Can you work these out from the model? Positions are in its coordinate system, mm. A direction names the side the tool comes from. Give positions to 0.01 mm unless a question says otherwise; leave off trailing zeros. Loops run counter-clockwise (first coordinate to the right, second up) from the corner with the lowest first, then second, coordinate; pieces in that order, holes last. Notation, with made-up numbers: M -38,46 L -3,46 A9 cw -3,54 Z; hole C -1.75,63 d11. An arc over 180 degrees is marked long. One line per item, written item: value. Start each with the question number.
from build123d import *

# Parameters (mm, degrees)
PAD_DEPTH    = 0.8
PAD001_DEPTH = 10
SKETCH003_R  = 3
PAD002_DEPTH = 6
POCKET_DEPTH = 5


with BuildPart() as part:
    # Sketch → Pad (new body)
    with BuildSketch(Plane.XZ):
        with BuildLine():
            Line((-25.5, 14.5), (-25.5, 48))
            ThreePointArc((-21.5, 52), (-24.328427, 50.828427), (-25.5, 48))
            Line((-21.5, 52), (21.5, 52))
            ThreePointArc((25.5, 48), (24.328427, 50.828427), (21.5, 52))
            Line((25.5, 48), (25.5, 14.5))
            Line((25.5, 14.5), (15.5, 14.5))
            Line((15.5, 14.5), (15.5, 24))
            Line((15.5, 24), (-15.5, 24))
            Line((-15.5, 24), (-15.5, 14.5))
            Line((-15.5, 14.5), (-25.5, 14.5))
        make_face()
    extrude(amount=PAD_DEPTH)

    # Sketch001 → Pad001 (join, symmetric)
    with BuildSketch(Plane.YZ):
        Polygon((-2, 24), (-9.7, 31.7), (-9.7, 32.5), (0, 32.5), (0, 24), align=None)
    extrude(amount=PAD001_DEPTH, both=True)

    # Sketch003 (on Face12 of Pad001) → Pad002 (join)
    with BuildSketch(Plane(origin=(0, 0, 32.5), x_dir=(-1, 0, 0), z_dir=(0, 0, 1))):
        with Locations((0, 5.5)):
            Circle(SKETCH003_R)
    extrude(amount=-PAD002_DEPTH)

    # Sketch004 (on Face5 of Pad002) → Pocket (cut)
    with BuildSketch(Plane.XZ.offset(0.8)):
        with BuildLine():
            Line((-12, 38.8), (-12, 46.8))
            Line((-12, 46.8), (-8, 46.8))
            Line((-8, 46.8), (-8, 38.8))
            ThreePointArc((-8, 38.8), (-7, 37.8), (-6, 38.8))
            Line((-6, 38.8), (-6, 48))
            Line((-6, 48), (-14, 48))
            Line((-14, 48), (-14, 38.8))
            ThreePointArc((-14, 38.8), (-13, 37.8), (-12, 38.8))
        make_face()
        with BuildLine():
            Line((12, 38.8), (12, 46.8))
            Line((12, 46.8), (8, 46.8))
            Line((8, 46.8), (8, 38.8))
            ThreePointArc((6, 38.8), (7, 37.8), (8, 38.8))
            Line((6, 38.8), (6, 48))
            Line((6, 48), (14, 48))
            Line((14, 48), (14, 38.8))
            ThreePointArc((12, 38.8), (13, 37.8), (14, 38.8))
        make_face()
    extrude(amount=-POCKET_DEPTH, mode=Mode.SUBTRACT)


solid = part.part
Q1. If we section it at A-A, the plane z = 45.5: Write out the boundary of the cut face in (x, y).
Q2. If we mould it in two halves opening along X, with no side actions, what happens to faces 5 (the face through (-24.297, -0.394, 50.859)), 6 (the face through (10, -4, 29)), 7 (the face through (7, -0.4, 37.8))? For each: released by +X, released by -X, zero draft, split by the parting line, or undercut.
Q3. If we section it at C-C, the plane y = -5.5: Write out the boundary of the cut face in (x, z), plus the area to 3 significant figures.
Q4. If we section it at D-D, the plane x = 0: Write out the boundary of the cut face in (y, z).
Q5. For P1, Ø1.5, axis at x = -13, y = -2, coming from the +Z side; P2, Ø4.5, axis at x = -1, y = -5, coming from the +Z side; P3, Ø4.5, axis at x = 1.5, y = -5.5, coming from the -Z side; P4, Ø2.5, axis at y = -6.5, z = 28, coming from the -X side, each with a flat end and sliding along its axis, tell me the tip position at first contact or that it passes through.
Q6. Which directions (+Z, -Z, +X, -X, +Y, -Y) give clear straight access to the entire face, cutting with the end or side of a thin tool? Please do faces 1 (the face through (0, -5, 32.5)), 2 (the face through (0, -6, 26.5)), 3 (the face through (-7, -0.4, 37.8)), 4 (the face through (-10, -4, 29)).
Q7. I need wall thicknesses on line 1 along Y through (x, z) = (2, 42); line 2 along X through (y, z) = (-5.75, 30); line 3 along Z through (x, y) = (-0.5, -7.5). Which ranges of each line are inside material? Lowest first, please.
Q8. If we section it at B-B, the plane x = -13: Write out the boundary of the cut face in (y, z).
Response:
1. outline: M -25.5,-0.8 L -14,-0.8 L -14,0 L -25.5,0 Z; M -12,-0.8 L -8,-0.8 L -8,0 L -12,0 Z; M -6,-0.8 L 6,-0.8 L 6,0 L -6,0 Z; M 8,-0.8 L 12,-0.8 L 12,0 L 8,0 Z; M 14,-0.8 L 25.5,-0.8 L 25.5,0 L 14,0 Z
2. face 5: released by -X
2. face 6: released by +X
2. face 7: undercut
3. outline: M -10,27.5 L -3,27.5 L -3,26.5 L 3,26.5 L 3,27.5 L 10,27.5 L 10,32.5 L -10,32.5 Z
3. area: 106 mm^2
4. outline: M -9.7,31.7 L -8.5,30.5 L -8.5,26.5 L -4.5,26.5 L -2,24 L 0,24 L 0,52 L -0.8,52 L -0.8,32.5 L -9.7,32.5 Z
5. P1: through
5. P2: z = 32.5
5. P3: z = 25.25
5. P4: x = -10
6. face 1: +Z, +X, -X, -Y
6. face 2: -Z, +X, -X, -Y
6. face 3: +Y, -Y
6. face 4: +Z, -Z, -X, -Y
7. line 1: -0.8 to 0
7. line 2: -10 to 10
7. line 3: 26.5 to 32.5
8. outline: M -0.8,24 L 0,24 L 0,37.8 L -0.8,37.8 Z; M -0.8,48 L 0,48 L 0,52 L -0.8,52 Z
